from build123d import *

# Parameters (mm, degrees)
BOSS_EXTRUDE1_DEPTH = 2
BOSS_EXTRUDE3_DEPTH = 6
SKETCH7_W           = 80.2
SKETCH7_H           = 2
BOSS_EXTRUDE4_DEPTH = 18.2
BOSS_EXTRUDE5_DEPTH = 2


with BuildPart() as part:
    # Sketch1 → Boss-Extrude1 (new body)
    with BuildSketch(Plane(origin=(0, 0, 0), x_dir=(1, 0, 0), z_dir=(0, 1, 0))):
        Polygon((0, 0), (30.4, 0), (30.4, 95.9), (18.2, 95.9), (18.2, 15.7), (0, 15.7), align=None)
    extrude(amount=BOSS_EXTRUDE1_DEPTH)

    # Sketch4 → Boss-Extrude3 (add)
    with BuildSketch(Plane(origin=(0, 2, 0), x_dir=(1, 0, 0), z_dir=(0, 1, 0))):
        Polygon((0, -2), (0, 0), (30.4, 0), (30.4, 95.9), (32.4, 95.9), (32.4, 0), (32.4, -2), align=None)
    extrude(amount=-BOSS_EXTRUDE3_DEPTH)

    # Sketch7 → Boss-Extrude4 (add)
    with BuildSketch(Plane.ZY.offset(-18.2)):
        with Locations((-55.8, 1)):
            Rectangle(SKETCH7_W, SKETCH7_H)
    extrude(amount=BOSS_EXTRUDE4_DEPTH)

    # Sketch8 → Boss-Extrude5 (add)
    with BuildSketch(Plane(origin=(0, 0, 0), x_dir=(-1, 0, 0), z_dir=(0, -1, 0))):
        Polygon((-5, 95.9), (0, 95.9), (0, 102.1), (-32.4, 102.1), (-32.4, 99.1), (-5, 99.1), align=None)
    extrude(amount=-BOSS_EXTRUDE5_DEPTH)


solid = part.part
For this review, take the finished solid that the model builds, in its own axes (mm). A direction names the side the tool comes from. Round coordinates to 2 decimals unless told otherwise and drop trailing zeros. Loops run counter-clockwise (first coordinate to the right, second up) from the corner with the lowest first, then second, coordinate; pieces in that order, holes last. Notation, with made-up numbers: (-38, 81.25) - (-4, 81.25) arc R22 ccw to (-4, 117.25) - close; hole circle Ø9 at (-39, -29). An arc over 180 degrees is marked (long way). Use one line per item in the form item = value.
1) We need section A-A on x = 16. Write out the cut boundary in (y, z).
Solutions:
outline = (-4, 0) - (0, 0) - (0, -95.9) - (2, -95.9) - (2, 2) - (-4, 2) - close; (0, -102.1) - (2, -102.1) - (2, -99.1) - (0, -99.1) - close
2) Mouldability with a two-part tool opening along Z and no side actions: class faces 4 (the face through (19, 1, -99.1)), 5 (the face through (16, 1, -102.1)), 6 (the face through (30.4, -2, -47)) as pulls with the +Z half, pulls with the -Z half, needs draft (parallel to the pull), parting line crosses it, or undercut.
Solutions:
face_4 = undercut
face_5 = pulls with the -Z half
face_6 = needs draft
3) Wall thickness on probe 1 along Z at (x, y) = (18.5, 1.5); probe 2 along X at (y, z) = (-3.2, -68); probe 3 along Z at (x, y) = (20, -2.6): over which ranges is each line inside the solid? List them lowest first.
Solutions:
probe_1 = -102.1 to -99.1, -95.9 to 2
probe_2 = 30.4 to 32.4
probe_3 = 0 to 2
4) Clearance check with flat-ended pins moving along their axes: P1, Ø2, axis at y = -2.5, z = -55.5, coming from the -X side; P2, Ø3, axis at x = 12.5, y = -3, coming from the -Z side; P3, Ø2, axis at y = 1, z = -98, coming from the +X side. State where each tip first meets the part, or that it passes through.
Solutions:
P1 = 30.4
P2 = 0
P3 = 5
5) We need section B-B on y = -0.9. Write out the cut boundary in (x, z), then the cut area to 3 significant figures.
Solutions:
outline = (0, 0) - (30.4, 0) - (30.4, -95.9) - (32.4, -95.9) - (32.4, 2) - (0, 2) - close
area = 257 mm2
6) Tool access review of faces 1 (the face through (21.9, 0.3, -95.9)), 2 (the face through (0, 1, -46)), 3 (the face through (15, -2, 0)): name each direction out of +Z, -Z, +X, -X, +Y, -Y from which nothing blocks a thin tool from reaching the whole face with its end or side.
Solutions:
face_1 = +X, +Y, -Y
face_2 = +Z, -Z, -X, +Y, -Y
face_3 = -Z, -X, -Y
7) We need section C-C on z = -72. Write out the cut boundary in (x, y), then the cut area to 3 significant figures.
Solutions:
outline = (0, 0) - (30.4, 0) - (30.4, -4) - (32.4, -4) - (32.4, 2) - (0, 2) - close
area = 72.8 mm2
